Geometry: see drawing. Coordinates: mm, zero at the bounding-box minimum. Give positions to 0.01 mm unless a question says otherwise; leave off trailing zeros. Order: outer loops, then holes, each group sorted by start corner. A loop starts at its lowest first (then second) coordinate and runs counter-clockwise, first axis right, second up. Notation, with made-up numbers: M 19,48.5 L 74,48.5 A20 ccw 74,86.5 Z; hole C 28.5,63 d1. An arc over 180 degrees is marked long. Use a Markdown table: item, result.
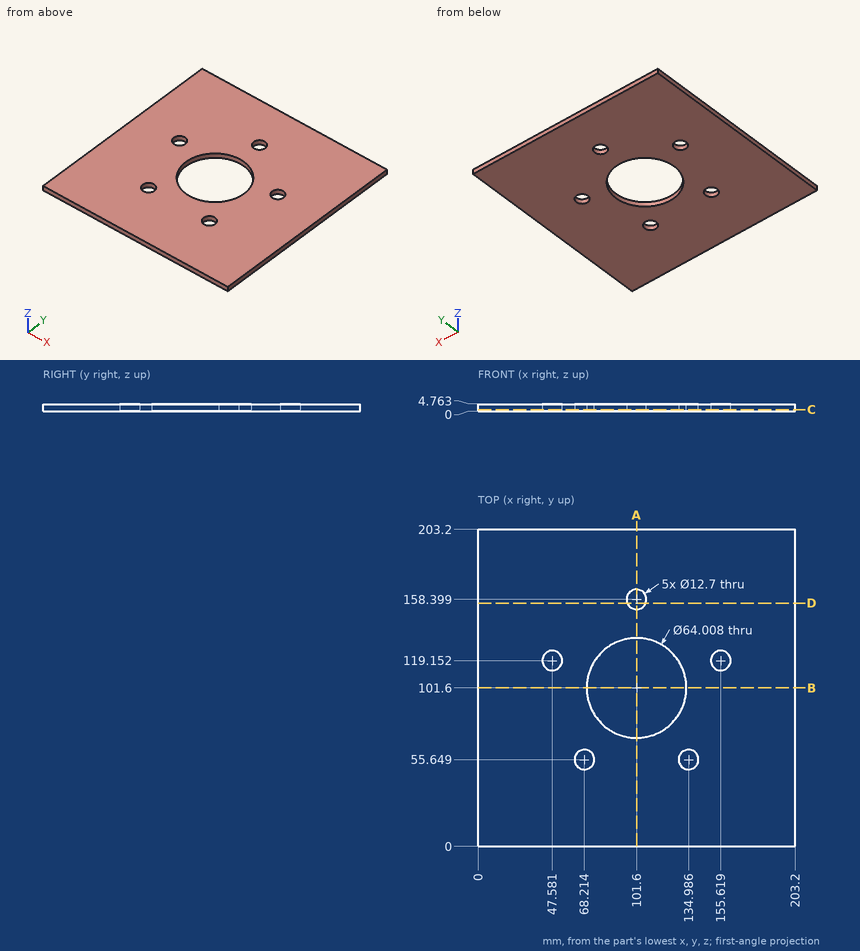
1) First-contact query: pin 1 Ø7.5 at (x, y) = (47.58, 119.15) entering from -Z. Flat tip, straight axial feed; report the tip coordinate or a pass-through.
Response values:
| item | result |
|---|---|
| pin 1 | passes through |
2) Cut plane B-B on y = 101.6. Return loops of the section in (x, z) (1 decimal), and give its area (3 significant figures).
Response values:
| item | result |
|---|---|
| outline | M 0,0 L 69.6,0 L 69.6,4.8 L 0,4.8 Z; M 133.6,0 L 203.2,0 L 203.2,4.8 L 133.6,4.8 Z |
| area | 663 mm² |
3) Material intervals for line 1 (X direction, y = 56, z = 3.4) (1 decimal); line 2 (Y direction, x = 101.6, z = 3.5) (1 decimal); line 3 (Y direction, x = 99.5, z = 1.85) (1 decimal), sorted ascending. Write a range as from..to.
Response values:
| item | result |
|---|---|
| line 1 | x = 0..61.9, 74.6..128.6, 141.3..203.2 |
| line 2 | y = 0..69.6, 133.6..152, 164.7..203.2 |
| line 3 | y = 0..69.7, 133.5..152.4, 164.4..203.2 |
4) Cut plane A-A on x = 101.6. Return loops of the section in (y, z) (1 decimal).
Response values:
| item | result |
|---|---|
| outline | M 0,0 L 69.6,0 L 69.6,4.8 L 0,4.8 Z; M 133.6,0 L 152,0 L 152,4.8 L 133.6,4.8 Z; M 164.7,0 L 203.2,0 L 203.2,4.8 L 164.7,4.8 Z |
5) Cut plane D-D on y = 156. Return loops of the section in (x, z).
Response values:
| item | result |
|---|---|
| outline | M 0,0 L 95.72,0 L 95.72,4.76 L 0,4.76 Z; M 107.48,0 L 203.2,0 L 203.2,4.76 L 107.48,4.76 Z |
6) Cut plane C-C on z = 1.1. State how many separate pieces and enclosed holes the cut face has, and give its area (3 significant figures).
Response values:
| item | result |
|---|---|
| separate pieces | 1 |
| enclosed holes | 6 |
| area | 37,400 mm² |
